The listing builds one solid part. Answer for the finished solid, in the listing's coordinates (mm). Face numbers are marked on the shaded views. A direction names the side the tool comes from. Coordinates: 2 decimals unless noted, no trailing zeros. Order: outer loops, then holes, each group sorted by start corner. A loop starts at its lowest first (then second) coordinate and runs counter-clockwise, first axis right, second up. Notation, with made-up numbers: (48.5, -24) -> (71.5, -24) arc R6 ccw to (71.5, -20) -> close; hole circle Ø11 at (11.25, -5.75). An arc over 180 degrees is marked (long way). Return JSON: item names as keys, results as strings.
from build123d import *

# Parameters (mm, degrees)
SKIZZE1_W                       = 70
SKIZZE1_H                       = 30
AUFSATZ_LINEAR_AUSTRAGEN1_DEPTH = 100
SCHNITT_LINEAR_AUSTRAGEN2_DEPTH = 126.6980509
SCHNITT_LINEAR_AUSTRAGEN3_DEPTH = 100
SCHNITT_LINEAR_AUSTRAGEN4_DEPTH = 126.6980509
WANDUNG1_T                      = -2
SKIZZE10_R                      = 3
AUFSATZ_LINEAR_AUSTRAGEN2_DEPTH = 2
SKIZZE12_R                      = 2
AUFSATZ_LINEAR_AUSTRAGEN3_DEPTH = 5
SKIZZE13_R                      = 1.5
SCHNITT_LINEAR_AUSTRAGEN5_DEPTH = 124.385574521
SKIZZE15_R                      = 2
SCHNITT_LINEAR_AUSTRAGEN6_DEPTH = 3
SKIZZE26_W                      = 26
SKIZZE26_H                      = 8
AUFSATZ_LINEAR_AUSTRAGEN4_DEPTH = 30
SKIZZE27_W                      = 24
SKIZZE27_H                      = 6
SCHNITT_LINEAR_AUSTRAGEN8_DEPTH = 28
SCHNITT_LINEAR_AUSTRAGEN9_REACH = 127.698
SKIZZE28_W                      = 9
SKIZZE28_H                      = 4


with BuildPart() as part:
    # Skizze1 → Aufsatz-Linear austragen1 (new body)
    with BuildSketch(Plane.XY):
        with Locations((35, 15)):
            Rectangle(SKIZZE1_W, SKIZZE1_H)
    extrude(amount=AUFSATZ_LINEAR_AUSTRAGEN1_DEPTH)

    # Skizze4 → Schnitt-Linear austragen2 (cut, through all)
    with BuildSketch(Plane(origin=(70, 0, 0), x_dir=(0, 0, -1), z_dir=(1, 0, 0))):
        Polygon((0, 15), (-20, 30), (0, 30), align=None)
    extrude(amount=-SCHNITT_LINEAR_AUSTRAGEN2_DEPTH, mode=Mode.SUBTRACT)

    # Skizze5 → Schnitt-Linear austragen3 (cut)
    with BuildSketch(Plane.XY.offset(100)):
        Polygon((0, 30), (20, 30), (0, 15), align=None)
        Polygon((70, 30), (50, 30), (70, 15), align=None)
    extrude(amount=-SCHNITT_LINEAR_AUSTRAGEN3_DEPTH, mode=Mode.SUBTRACT)

    # Skizze8 → Schnitt-Linear austragen4 (cut, through all)
    with BuildSketch(Plane(origin=(70, 0, 0), x_dir=(0, 0, -1), z_dir=(1, 0, 0))):
        Polygon((-100, 30), (-100, 15), (-85, 21), (-40, 21), (-34, 30), align=None)
    extrude(amount=-SCHNITT_LINEAR_AUSTRAGEN4_DEPTH, mode=Mode.SUBTRACT)

    # Wandung1
    wandung1_openings = [part.faces().sort_by_distance(p)[0] for p in [
        (35, 0, 50),
    ]]
    offset(amount=WANDUNG1_T, openings=wandung1_openings, kind=Kind.INTERSECTION)

    # Skizze10 → Aufsatz-Linear austragen2 (add)
    with BuildSketch(Plane.XZ.offset(-19)):
        with Locations(Location((35, 79.614835193, 0), (0, 0, 270))):
            Circle(SKIZZE10_R)
    extrude(amount=AUFSATZ_LINEAR_AUSTRAGEN2_DEPTH)

    # Skizze12 → Aufsatz-Linear austragen3 (add)
    with BuildSketch(Plane.XZ.offset(-17)):
        with Locations(Location((35, 79.614835193, 0), (0, 0, 270))):
            Circle(SKIZZE12_R)
    extrude(amount=AUFSATZ_LINEAR_AUSTRAGEN3_DEPTH)

    # Skizze13 → Schnitt-Linear austragen5 (cut, through all)
    with BuildSketch(Plane.XZ.offset(-12)):
        with Locations(Location((35, 79.614835193, 0), (0, 0, 270))):
            Circle(SKIZZE13_R)
    extrude(amount=-SCHNITT_LINEAR_AUSTRAGEN5_DEPTH, mode=Mode.SUBTRACT)

    # Skizze15 → Schnitt-Linear austragen6 (cut)
    with BuildSketch(Plane(origin=(0, 21, 0), x_dir=(1, 0, 0), z_dir=(0, 1, 0))):
        with Locations(Location((35, -79.614835193, 0), (0, 0, 90))):
            Circle(SKIZZE15_R)
    extrude(amount=-SCHNITT_LINEAR_AUSTRAGEN6_DEPTH, mode=Mode.SUBTRACT)

    # Skizze26 → Aufsatz-Linear austragen4 (add)
    with BuildSketch(Plane(origin=(0, 30, 0), x_dir=(1, 0, 0), z_dir=(0, 1, 0))):
        with Locations((35, -27)):
            Rectangle(SKIZZE26_W, SKIZZE26_H)
    extrude(amount=-AUFSATZ_LINEAR_AUSTRAGEN4_DEPTH)

    # Skizze27 → Schnitt-Linear austragen8 (cut)
    with BuildSketch(Plane(origin=(0, 30, 0), x_dir=(1, 0, 0), z_dir=(0, 1, 0))):
        with Locations((35, -27)):
            Rectangle(SKIZZE27_W, SKIZZE27_H)
    extrude(amount=-SCHNITT_LINEAR_AUSTRAGEN8_DEPTH, mode=Mode.SUBTRACT)

    # Skizze28 → Schnitt-Linear austragen9 (cut, up to next)
    with BuildSketch(Plane.XZ, mode=Mode.PRIVATE) as schnitt_linear_austragen9_sk1:
        with Locations((41.5, 27)):
            Rectangle(SKIZZE28_W, SKIZZE28_H)
    schnitt_linear_austragen9_tool1 = extrude(schnitt_linear_austragen9_sk1.sketch, amount=-SCHNITT_LINEAR_AUSTRAGEN9_REACH, mode=Mode.PRIVATE) & part.part
    add(schnitt_linear_austragen9_tool1.solids().sort_by_distance((41.5, 0, 27))[0], mode=Mode.SUBTRACT)


solid = part.part
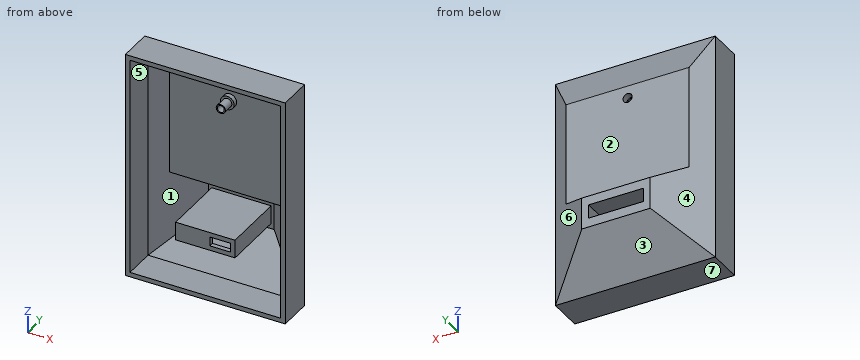
1. For the marked faces 1, 2 and 3, determine the directions among +Z, -Z, +X, -X, +Y, -Y from which every point of the face is accessible in a straight line to the end or side of a thin tool.
Answer block:
{"face 1": "-Y", "face 2": "+Z, +X, -X, +Y", "face 3": "-Z, +X, -X, +Y"}
2. Consider line 1 (Z direction, x = 23, y = 1.5); line 2 (X direction, y = 1.75, z = 73); line 3 (Z direction, x = 62, y = 10). Determine where each line is inside the solid, lowest interval first. Write a range as from..to.
Answer block:
{"line 1": "z = 0..2, 23..31, 98..100", "line 2": "x = 0..2, 68..70", "line 3": "z = 0..2, 98..100"}
3. The part is cut by section A-A on y = 7. Give the vertices of the cut face in (x, z), and give its area (3 significant figures).
Answer block:
{"outline": "(0, 0) -> (70, 0) -> (70, 100) -> (0, 100) -> close; (22, 23) -> (48, 23) -> (48, 31) -> (22, 31) -> close; hole (2, 2) -> (68, 2) -> (68, 98) -> (2, 98) -> close; hole (23, 24) -> (47, 24) -> (47, 30) -> (23, 30) -> close", "area": "728 mm2"}
4. Each of these flat-tipped pins is pushed along its axis until it touches: pin 1 Ø8 at (x, z) = (56, 22.5) entering from +Y; pin 2 Ø8 at (x, z) = (52, 18) entering from -Y; pin 3 Ø3 at (x, z) = (34, 79) entering from -Y; pin 4 Ø1.2 at (x, z) = (34.5, 79.5) entering from +Y. Where does it stop, or does it pass through?
Answer block:
{"pin 1": "stops at y = 28.5", "pin 2": "stops at y = 23", "pin 3": "stops at y = 12", "pin 4": "passes through"}
5. The part is cut by section C-C on x = 57. Give the vertices of the cut face in (y, z), and give its area (3 significant figures).
Answer block:
{"outline": "(0, 0) -> (15, 0) -> (24.75, 13) -> (24.75, 37.5) -> (21, 40) -> (21, 85) -> (15, 100) -> (0, 100) -> (0, 98) -> (13.65, 98) -> (19, 84.61) -> (19, 38.93) -> (22.25, 36.76) -> (22.25, 13) -> (14, 2) -> (0, 2) -> close", "area": "278 mm2"}
6. The part is cut by section D-D on y = 23. Give the vertices of the cut face in (x, z).
Answer block:
{"outline": "(10.67, 10.67) -> (59.33, 10.67) -> (59.33, 38.67) -> (10.67, 38.67) -> close; (22, 23) -> (48, 23) -> (48, 31) -> (22, 31) -> close; hole (14, 14) -> (56, 14) -> (56, 36.26) -> (14, 36.26) -> close; hole (23, 24) -> (47, 24) -> (47, 30) -> (23, 30) -> close"}
7. The part is cut by section B-B on z = 50. Give the vertices of the cut face in (x, y).
Answer block:
{"outline": "(0, 0) -> (2, 0) -> (2, 14) -> (8.67, 19) -> (61.33, 19) -> (68, 14) -> (68, 0) -> (70, 0) -> (70, 15) -> (62, 21) -> (8, 21) -> (0, 15) -> close"}
8. Determine the mould class of the marked faces 4, 5, 6 and 7 for opening direction X: pulls with the +X half, pulls with the -X half, needs draft (parallel to the pull), parting line crosses it, or undercut.
Answer block:
{"face 4": "pulls with the -X half", "face 5": "undercut", "face 6": "pulls with the +X half", "face 7": "needs draft"}
